Autodesk Inventor part; units mm, degrees
ref_plane "Work Plane1" through (0, 0, -60) normal (0, 0, 1) x (1, 0, 0)
ref_plane "YZ Plane" through (0, 0, 0) normal (1, 0, 0) x (0, 1, 0)
ref_plane "XZ Plane" through (0, 0, 0) normal (0, 1, 0) x (-1, 0, 0)
sketch "Sketch1" plane through (0, 0, 0) normal (0, 0, 1) x (1, 0, 0)
  arc A0 (-20.5913, 51) -> (20.5913, 51) centre (0, 0) ccw
  circle A1 centre (0, 0) radius 50
  line L0 (-40.5, 55) -> (40.5, 55)
  arc A2 (-40.5, 55) -> (-40.5, 51) centre (-40.5, 53) ccw
  arc A3 (40.5, 51) -> (40.5, 55) centre (40.5, 53) ccw
  line L1 (40.5, 51) -> (19.5959, 51)
  line L2 (40.5, 51) -> (19.5959, 51)
  line L3 (40.5, 51) -> (19.5959, 51)
  line L4 (19.5959, 51) -> (-40.5, 51)
  line L5 (0, 51) -> (0, 50)
  dimension "d0" = 110
  dimension "d1" = 100
extrude "Extrusion1" add sketch "Sketch1" against normal blind 120
sketch "Sketch2" plane through (0, 0, 0) normal (0, 0, 1) x (1, 0, 0)
  circle A0 centre (0, 0) radius 50
  line L0 (-40.5, 51) -> (-20.5913, 51)
  arc A1 (-20.5913, 51) -> (20.5913, 51) centre (0, 0) ccw
  line L1 (20.5913, 51) -> (40.5, 51)
  arc A2 (40.5, 51) -> (40.5, 55) centre (40.5, 53) ccw
  line L2 (40.5, 55) -> (-40.5, 55)
  arc A3 (-40.5, 55) -> (-40.5, 51) centre (-40.5, 53) ccw
  circle A4 centre (0, 0) radius 55
  point P0 (160.5446, 51)
extrude "Extrusion2" cut sketch "Sketch2" against normal blind 30 contours A3 L2 A4 L0 | L2 A2 L1 A4
ref_plane "Work Plane1" through (0, 0, -60) normal (0, 0, 1) x (1, 0, 0)
sketch "Sketch3" plane through (50, 55, 0) normal (0, 1, 0) x (1, 0, 0)
  line L0 (-44, 120) -> (-56, 120)
  line L1 (-30.4041, 0) -> (-69.5959, 0)
  line L2 (-56, 120) -> (-44, 120)
  line L3 (-44, 120) -> (-44, 95)
  line L4 (-48, 91) -> (-52, 91)
  line L5 (-56, 95) -> (-56, 120)
  arc A0 (-56, 95) -> (-52, 91) centre (-52, 95) ccw
  arc A1 (-48, 91) -> (-44, 95) centre (-48, 95) ccw
  point P0 (17.7764, 120)
  point P1 (-44, 91)
  point P2 (-56, 91)
  dimension "d33" = 12
  dimension "d43" = 12
  dimension "d44" = 29
  dimension "d45" = 4
extrude "Extrusion3" cut sketch "Sketch3" against normal blind 7
mirror "Mirror2" about plane through (0, 0, -60) normal (0, 0, 1) of "Extrusion2"
fillet "Fillet1" radius 4 2 edges at (-6, 52.1552, -120) (6, 52.1552, -120)
sketch "Sketch4" plane through (-40.5, 55, -30) normal (0, 1, 0) x (1, 0, 0)
  line L0 (40.5, 60) -> (0, 60)
  line L1 (0, 0) -> (0, 60)
  line L2 (0, 0) -> (40.5, 0)
  line L3 (40.5, 0) -> (81, 0)
  line L4 (81, 0) -> (81, 60)
  line L5 (81, 60) -> (40.5, 60)
  line L6 (81, 0) -> (81, 60)
  line L7 (19.9087, 60) -> (19.9087, 0)
  line L8 (61.0913, 0) -> (61.0913, 60)
  line L9 (81, 0) -> (61.0913, 0)
  circle A0 centre (6.9544, 30) radius 3
  circle A1 centre (74.0456, 30) radius 3
  point P0 (40.5, -30)
  dimension "d48" = 6
  dimension "d51" = 6
extrude "Extrusion4" cut sketch "Sketch4" against normal blind 5 contours A0 | A1
properties part number "Propeller Shroud" material "ABS Plastic"
Design review of the part built by this model. Coordinates are the model's own, in mm. A direction names the side the tool comes from. Round coordinates to 2 decimals unless told otherwise and drop trailing zeros. Order: outer loops, then holes, each group sorted by start corner. A loop starts at its lowest first (then second) coordinate and runs counter-clockwise, first axis right, second up. Notation, with made-up numbers: (28, 27) - (71, 27) arc R28 cw to (71, 50) - close; hole circle Ø10 at (58.25, 8.25). An arc over 180 degrees is marked (long way). Return JSON: item names as keys, results as strings.
Q1. Wall thickness on L1, parallel to X at y = 0, z = -24; L2, parallel to X at y = 54, z = -60; L3, parallel to X at y = 53.3, z = -60: over which ranges is each line inside the solid? List them lowest first. Write a range as [from, to].
Computed values:
{"L1": "x = [-55, -50], [50, 55]", "L2": "x = [-42.23, -36.55], [-30.55, 30.55], [36.55, 42.23]", "L3": "x = [-42.48, -36.55], [-30.55, 30.55], [36.55, 42.48]"}
Q2. Consider section B-B on x = -38.5. Write out the cut boundary in (y, z).
Computed values:
{"outline": "(-39.28, -120) - (-31.9, -120) - (-31.9, 0) - (-39.28, 0) - close; (31.9, -120) - (39.28, -120) - (39.28, 0) - (31.9, 0) - close; (51, -90) - (55, -90) - (55, -30) - (51, -30) - close"}
Q3. Consider section A-A on z = -60. Write out the cut boundary in (x, y), plus the area to 3 significant figures.
Computed values:
{"outline": "(-40.5, 51) - (-36.55, 51) - (-36.55, 55) - (-40.5, 55) arc R2 ccw to start; (-30.55, 51) - (-20.59, 51) arc R55 ccw (long way) to (20.59, 51) - (30.55, 51) - (30.55, 55) - (-30.55, 55) - close; (36.55, 51) - (40.5, 51) arc R2 ccw to (40.5, 55) - (36.55, 55) - close; hole circle Ø100 at (0, 0)", "area": "1,830 mm2"}
Q4. The part is to be moulded in two halves that separate along Z. For faces 1 (the cylindrical face through (4.797, 52.338, -92.141)), 2 (the flat face through (-26, 53, -30)), 3 (the cylindrical face through (42.5, 53, -59.6)), say which applies: pulls with the +Z half, pulls with the -Z half, needs draft (parallel to the pull), parting line crosses it, or undercut.
Computed values:
{"face 1": "pulls with the -Z half", "face 2": "pulls with the +Z half", "face 3": "needs draft"}
Q5. Consider section C-C on y = 0. Write out the cut boundary in (x, z), plus the area to 3 significant figures.
Computed values:
{"outline": "(-55, -120) - (-50, -120) - (-50, 0) - (-55, 0) - close; (50, -120) - (55, -120) - (55, 0) - (50, 0) - close", "area": "1,200 mm2"}
Q6. Consider section D-D on z = -25. Write out the cut boundary in (x, y), plus the area to 3 significant figures.
Computed values:
{"outline": "circle Ø110 at (0, 0); hole circle Ø100 at (0, 0)", "area": "1,650 mm2"}
Q7. Machinability: for faces 4 (the cylindrical face through (7.141, 51.791, -118.797)), 5 (the flat face through (26, 53, -30)), 6 (the flat face through (-26, 53, -90)), which of the approach directions +Z, -Z, +X, -X, +Y, -Y give a long, thin tool a straight path to every point of the face, cutting with its end or side? Answer none if there is none.
Computed values:
{"face 4": "-Z, +Y", "face 5": "+Z, +X, +Y", "face 6": "-Z, -X, +Y"}
Q8. For pin 1 Ø5 at (x, z) = (-33.55, -60) entering from +Y; pin 2 Ø2.5 at (y, z) = (52, -105) entering from +X; pin 3 Ø8 at (y, z) = (-39.5, -104.5) entering from -X, all flat-tipped, find the tip position at first contact; note any pin that passes through.
Computed values:
{"pin 1": "stops at y = 45.4", "pin 2": "stops at x = 21.2", "pin 3": "stops at x = -42.01"}
